Work out the finished part from the listing and answer in its coordinate system (mm). A direction names the side the tool comes from. Give positions to 0.01 mm unless a question says otherwise; leave off trailing zeros. Loops run counter-clockwise (first coordinate to the right, second up) from the corner with the lowest first, then second, coordinate; pieces in that order, holes last. Notation, with made-up numbers: (50.5, 66.25) - (77.5, 66.25) arc R8 cw to (77.5, 73.25) - close; hole circle Ø1 at (-7.75, 13). An arc over 180 degrees is marked (long way). Use CSV: the item, a comma, the result in double quotes.
from build123d import *

# Parameters (mm, degrees)
SKETCH_W        = 73
SKETCH_H        = 48
PAD_DEPTH       = 24.5
SKETCH001_W     = 70
SKETCH001_H     = 45
POCKET_DEPTH    = 23
FILLET_R        = 1
FILLET001_R     = 1
FILLET002_R     = 1
FILLET003_R     = 1
SKETCH002_W     = 4
SKETCH002_H     = 4
PAD001_DEPTH    = 5
FILLET004_R     = 1
SKETCH003_W     = 4
SKETCH003_H     = 4
PAD002_DEPTH    = 5
SKETCH004_R     = 1.4
POCKET001_DEPTH = 5
FILLET005_R     = 1
FILLET006_R     = 1
SKETCH005_R     = 1.4
POCKET002_DEPTH = 5
FILLET007_R     = 1
SKETCH006_R     = 1.4
POCKET003_DEPTH = 5
SKETCH007_R     = 16
POCKET004_DEPTH = 5
SKETCH008_R     = 4
POCKET005_DEPTH = 5


with BuildPart() as part:
    # Sketch → Pad (new body)
    with BuildSketch(Plane.XY):
        with Locations((36.5, 24)):
            Rectangle(SKETCH_W, SKETCH_H)
    extrude(amount=PAD_DEPTH)

    # Sketch001 (on Face6 of Pad) → Pocket (cut)
    with BuildSketch(Plane.XY.offset(24.5)):
        with Locations((36.5, 24)):
            Rectangle(SKETCH001_W, SKETCH001_H)
    extrude(amount=-POCKET_DEPTH, mode=Mode.SUBTRACT)

    # Fillet
    fillet_edges = [part.edges().sort_by_distance(p)[0] for p in [
        (73, 0, 12.25),
    ]]
    fillet(fillet_edges, radius=FILLET_R)

    # Fillet001
    fillet001_edges = [part.edges().sort_by_distance(p)[0] for p in [
        (73, 24.5, 0),
    ]]
    fillet(fillet001_edges, radius=FILLET001_R)

    # Fillet002
    fillet002_edges = [part.edges().sort_by_distance(p)[0] for p in [
        (36, 48, 0),
    ]]
    fillet(fillet002_edges, radius=FILLET002_R)

    # Fillet003
    fillet003_edges = [part.edges().sort_by_distance(p)[0] for p in [
        (0, 24, 0),
    ]]
    fillet(fillet003_edges, radius=FILLET003_R)

    # Sketch002 (on Face1 of Fillet003) → Pad001 (join)
    with BuildSketch(Plane.XY.offset(24.5)):
        with Locations((3.499952, 3.499965)):
            Rectangle(SKETCH002_W, SKETCH002_H)
    extrude(amount=-PAD001_DEPTH)

    # Fillet004
    fillet004_edges = [part.edges().sort_by_distance(p)[0] for p in [
        (5.499952, 5.499965, 22),
    ]]
    fillet(fillet004_edges, radius=FILLET004_R)

    # Sketch003 (on Face8 of Fillet004) → Pad002 (join)
    with BuildSketch(Plane.XY.offset(24.5)):
        with Locations((3.499993, 44.500004)):
            Rectangle(SKETCH003_W, SKETCH003_H)
        with Locations((69.500023, 44.500011)):
            Rectangle(SKETCH003_W, SKETCH003_H)
        with Locations((69.500008, 3.499997)):
            Rectangle(SKETCH003_W, SKETCH003_H)
    extrude(amount=-PAD002_DEPTH)

    # Sketch004 (on Face32 of Pad002) → Pocket001 (cut)
    with BuildSketch(Plane.XY.offset(24.5)):
        with Locations((3.503523, 44.499481)):
            Circle(SKETCH004_R)
        with Locations((69.500092, 44.497658)):
            Circle(SKETCH004_R)
    extrude(amount=-POCKET001_DEPTH, mode=Mode.SUBTRACT)

    # Fillet005
    fillet005_edges = [part.edges().sort_by_distance(p)[0] for p in [
        (67.500023, 42.500011, 22),
    ]]
    fillet(fillet005_edges, radius=FILLET005_R)

    # Fillet006
    fillet006_edges = [part.edges().sort_by_distance(p)[0] for p in [
        (5.499993, 42.500004, 22),
    ]]
    fillet(fillet006_edges, radius=FILLET006_R)

    # Sketch005 (on Face45 of Fillet006) → Pocket002 (cut)
    with BuildSketch(Plane.XY.offset(24.5)):
        with Locations((69.49865, 3.49611)):
            Circle(SKETCH005_R)
    extrude(amount=-POCKET002_DEPTH, mode=Mode.SUBTRACT)

    # Fillet007
    fillet007_edges = [part.edges().sort_by_distance(p)[0] for p in [
        (67.500008, 5.499997, 22),
    ]]
    fillet(fillet007_edges, radius=FILLET007_R)

    # Sketch006 (on Face35 of Fillet007) → Pocket003 (cut)
    with BuildSketch(Plane.XY.offset(24.5)):
        with Locations((3.5, 3.5)):
            Circle(SKETCH006_R)
    extrude(amount=-POCKET003_DEPTH, mode=Mode.SUBTRACT)

    # Sketch007 (on Face51 of Pocket003) → Pocket004 (cut)
    with BuildSketch(Plane(origin=(0, 0, 0), x_dir=(1, 0, 0), z_dir=(0, 0, -1))):
        with Locations((49.750546, -24)):
            Circle(SKETCH007_R)
    extrude(amount=-POCKET004_DEPTH, mode=Mode.SUBTRACT)

    # Sketch008 (on Face21 of Pocket004) → Pocket005 (cut)
    with BuildSketch(Plane(origin=(0, 0, 0), x_dir=(0, -1, 0), z_dir=(-1, 0, 0))):
        with Locations((-10.616032, 17.928658)):
            Circle(SKETCH008_R)
    extrude(amount=-POCKET005_DEPTH, mode=Mode.SUBTRACT)


solid = part.part
Item 1: A cutting plane is placed at A-A on x = 3.5. Determine the outline of the cut face in (y, z), and give its area (3 significant figures).
Determined:
outline,"(0, 1) arc R1 ccw to (1, 0) - (47, 0) arc R1 ccw to (48, 1) - (48, 24.5) - (45.9, 24.5) - (45.9, 19.5) - (46.5, 19.5) - (46.5, 1.5) - (1.5, 1.5) - (1.5, 19.5) - (2.1, 19.5) - (2.1, 24.5) - (0, 24.5) - close; (4.9, 19.5) - (5.5, 19.5) - (5.5, 24.5) - (4.9, 24.5) - close; (42.5, 19.5) - (43.1, 19.5) - (43.1, 24.5) - (42.5, 24.5) - close"
area,"153 mm²"
Item 2: A cutting plane is placed at B-B on y = 24. Determine the outline of the cut face in (x, z).
Determined:
outline,"(0, 1) arc R1 ccw to (1, 0) - (33.75, 0) - (33.75, 1.5) - (1.5, 1.5) - (1.5, 24.5) - (0, 24.5) - close; (65.75, 0) - (72, 0) arc R1 ccw to (73, 1) - (73, 24.5) - (71.5, 24.5) - (71.5, 1.5) - (65.75, 1.5) - close"
Item 3: Find the intervals of material crossed by line 1 (X direction, y = 3.5, z = 7.75); line 2 (Y direction, x = 22, z = 15); line 3 (Z direction, x = 61, y = 35.5), in increasing order.
Determined:
line 1,"x = 0 to 1.5, 71.5 to 73"
line 2,"y = 0 to 1.5, 46.5 to 48"
line 3,"z = 0 to 1.5"
Item 4: A cutting plane is placed at D-D on x = 61. Determine the outline of the cut face in (y, z).
Determined:
outline,"(0, 1) arc R1 ccw to (1, 0) - (12.62, 0) - (12.62, 1.5) - (1.5, 1.5) - (1.5, 24.5) - (0, 24.5) - close; (35.38, 0) - (47, 0) arc R1 ccw to (48, 1) - (48, 24.5) - (46.5, 24.5) - (46.5, 1.5) - (35.38, 1.5) - close"
Item 5: A cutting plane is placed at C-C on z = 2.5. Determine the outline of the cut face in (x, y).
Determined:
outline,"(0, 1) arc R1 ccw to (1, 0) - (72, 0) arc R1 ccw to (73, 1) - (73, 47) arc R1 ccw to (72, 48) - (1, 48) arc R1 ccw to (0, 47) - close; hole (1.5, 1.5) - (71.5, 1.5) - (71.5, 46.5) - (1.5, 46.5) - close"
Item 6: The mould has two halves that part along Y. Classify faces 1 (the flat face through (28, 24, 0)), 2 (the flat face through (36, 48, 13)), 3 (the cylindrical face through (4.15, 2.26, 22.04)): pulls with the +Y half, pulls with the -Y half, needs draft (parallel to the pull), parting line crosses it, or undercut.
Determined:
face 1,"needs draft"
face 2,"pulls with the +Y half"
face 3,"undercut"
Item 7: Given P1, Ø13.5, axis at x = 24, y = 26, coming from the +Z side; P2, Ø13, axis at y = 10.62, z = 17.93, coming from the -X side, each flat-ended and moving along its own axis, determine where each tip first touches the part or whether it passes through.
Determined:
P1,"stops at z = 1.5"
P2,"stops at x = 0"
Item 8: For faces 4 (the flat face through (67.5, 3, 22)), 5 (the cylindrical face through (37.053, 33.736, 0.74)), 6 (the flat face through (2, 45, 19.5)), determine the directions among +Z, -Z, +X, -X, +Y, -Y from which every point of the face is accessible in a straight line to the end or side of a thin tool.
Determined:
face 4,"+Z"
face 5,"+Z, -Z"
face 6,"none"
